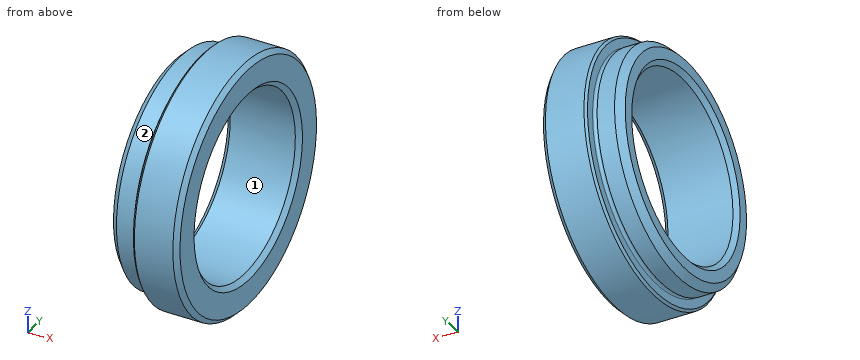
```python
from build123d import *


with BuildPart() as part:
    # Croquis2 → Revolución1 (revolve)
    with BuildSketch(Plane.XY, mode=Mode.PRIVATE) as revoluci_n1_sk:
        with BuildLine():
            Line((0, 23.5), (0, 21))
            Line((0, 21), (1, 20))
            Line((1, 20), (15.35, 20))
            Line((15.35, 20), (16.35, 21))
            Line((16.35, 21), (16.35, 26.45))
            Line((16.35, 26.45), (15.35, 27.45))
            Line((15.35, 27.45), (6.85, 27.45))
            Line((6.85, 27.45), (6.35, 26.95))
            Line((6.35, 26.95), (6.35, 25))
            ThreePointArc((6.35, 25), (5.85, 24.5), (5.35, 25))
            Line((5.35, 25), (1.5, 25))
            Line((1.5, 25), (0, 23.5))
        make_face()
    revolve(revoluci_n1_sk.sketch.rotate(Axis((0, 0, 0), (1, 0, 0)), 90), axis=Axis((0, 0, 0), (1, 0, 0)))


solid = part.part
```
Source: CAD feature listing. Evaluate the final solid. Frame: model axes, mm. Face numbers are marked on the shaded views. A direction names the side the tool comes from. Give positions to 0.01 mm unless a question says otherwise; leave off trailing zeros. Loops run counter-clockwise (first coordinate to the right, second up) from the corner with the lowest first, then second, coordinate; pieces in that order, holes last. Notation, with made-up numbers: (-32, -37) -> (-19, -37) arc R28 ccw to (-19, -3) -> close; hole circle Ø10 at (8.25, 89). An arc over 180 degrees is marked (long way). Put each result on its own line as item: value. Start each with the question number.
1) Reachability of the marked faces 1 and 2 from +Z, -Z, +X, -X, +Y, -Y: full face, straight path, thin tool, end or side. Return the list, or none.
2) Material intervals for probe 1 along Y at (x, z) = (7, 0); probe 2 along Z at (x, y) = (15, 13.5); probe 3 along Z at (x, y) = (2, -4.5), sorted ascending.
3) Cut plane A-A (y = 0). Return loops of the section in (x, z), then the cut area to 3 significant figures.
4) Contact query for flat-ended pins moving along their axis: P1, Ø4, axis at x = 4, y = -9, coming from the -Z side; P2, Ø1, axis at x = 9, z = 20.5, coming from the -Y side; P3, Ø3, axis at y = -15, z = -12, coming from the +X side. Output: stop coordinate, or through.
5) Cut plane C-C (x = 4). Return loops of the section in (y, z), then the cut area to 3 significant figures.
6) Cut plane D-D (x = 9.75). Return loops of the section in (y, z), then the cut area to 3 significant figures.
Results are:
1. face 1: +X, -X
1. face 2: -X
2. probe 1: y = -27.45 to -20, 20 to 27.45
2. probe 2: z = -23.9 to -14.76, 14.76 to 23.9
2. probe 3: z = -24.59 to -19.49, 19.49 to 24.59
3. outline: (0, -23.5) -> (1.5, -25) -> (5.35, -25) arc R0.5 cw to (6.35, -25) -> (6.35, -26.95) -> (6.85, -27.45) -> (15.35, -27.45) -> (16.35, -26.45) -> (16.35, -21) -> (15.35, -20) -> (1, -20) -> (0, -21) -> close; (0, 21) -> (1, 20) -> (15.35, 20) -> (16.35, 21) -> (16.35, 26.45) -> (15.35, 27.45) -> (6.85, 27.45) -> (6.35, 26.95) -> (6.35, 25) arc R0.5 cw to (5.35, 25) -> (1.5, 25) -> (0, 23.5) -> close
3. area: 206 mm2
4. P1: stops at z = -24
4. P2: stops at y = -18.8
4. P3: stops at x = 16.06
5. outline: circle Ø50 at (0, 0); hole circle Ø40 at (0, 0)
5. area: 707 mm2
6. outline: circle Ø54.9 at (0, 0); hole circle Ø40 at (0, 0)
6. area: 1,110 mm2
